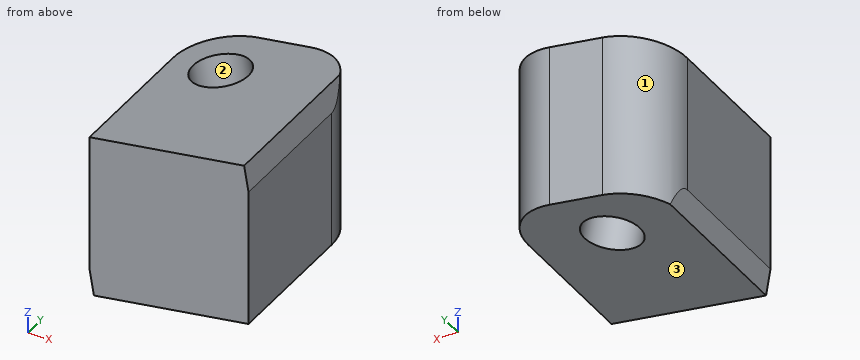
Autodesk Inventor part; units mm, degrees
ref_plane "YZ Plane" through (0, 0, 0) normal (1, 0, 0) x (0, 1, 0)
ref_plane "XZ Plane" through (0, 0, 0) normal (0, 1, 0) x (-1, 0, 0)
ref_plane "XY Plane" through (0, 0, 0) normal (0, 0, 1) x (1, 0, 0)
sketch "BaseSC" plane through (0, 0, 0) normal (0, 1, 0) x (-1, 0, 0)
  line L0 (15, 13) -> (-15, 13)
  line L1 (-15, 13) -> (-15, -13)
  line L2 (-15, -13) -> (15, -13)
  line L3 (15, -13) -> (15, 13)
  line L4 (15, 13) -> (-15, -13) construction
  line L5 (-15, 13) -> (15, -13) construction
  line L6 (15, 13) -> (14.1667, 17.9301)
  line L7 (14.1667, 17.9301) -> (-15, 13)
  line L8 (0, 0) -> (8.3423, 0)
  line L9 (15, -13) -> (14.1667, -17.9301)
  line L10 (14.1667, -17.9301) -> (-15, -13)
  line L11 (-15, 13) -> (-14.1667, 17.9301)
  line L12 (-14.1667, 17.9301) -> (15, 13)
  dimension "d0" = 30
  dimension "d1" = 26
  dimension "d9" = 5
  dimension "d10" = 90
  dimension "d17" = 5
  dimension "d18" = 90
sketch "スケッチ2" plane through (0, 0, 0) normal (0, 0, 1) x (1, 0, 0)
  point P0 (0, 0)
extrude "押し出し1" add sketch "BaseSC" against normal blind 30 contours L3 L2 L1 L0
sketch "スケッチ3" plane through (15, 0, 13) normal (1, 0, 0) x (0, 0, -1)
  line L0 (2.5, -1.5742) -> (23.5, -1.5742)
  line L1 (23.5, -1.5742) -> (23.5, -28.5742)
  line L2 (23.5, -28.5742) -> (2.5, -28.5742)
  line L3 (2.5, -28.5742) -> (2.5, -1.5742)
  line L4 (2.5, -1.5742) -> (23.5, -28.5742) construction
  line L5 (23.5, -1.5742) -> (2.5, -28.5742) construction
  ellipse E0 centre (13, -15.0742) end of major axis (23.5, -15.0742) minor radius 13.5
  point P0 (13, 0)
  dimension "d5" = 21
  dimension "d6" = 27
extrude "押し出し2" cut sketch "スケッチ3" against normal through all contours E0
extrude "押し出し3" add sketch "BaseSC" along normal blind 36 contours L3 L2 L1 L0 | L9 L10 L2
extrude "押し出し5" add sketch "BaseSC" along normal blind 36 contours L0 L7 L12 | L11 L12 L7
sketch "スケッチ5" plane through (-14.1667, 0, -17.9301) normal (0.1666667, 0, -0.9860133) x (-0.9860133, 0, -0.1666667)
  circle A0 centre (-14.1422, 25) radius 5.3
  line L0 (-29.5804, 0) -> (0, 0)
  point P0 (-16.9569, 0)
  dimension "d21" = 10.6
  dimension "d22" = 25
extrude "押し出し6" cut sketch "スケッチ5" against normal through all
sketch "スケッチ6" plane through (0, -30, 0) normal (0, -1, 0) x (1, 0, 0)
  line L0 (15, -1) -> (-15, -1)
  line L1 (-15, -1) -> (-15, 1)
  line L2 (-15, 1) -> (15, 1)
  line L3 (15, 1) -> (15, -1)
  line L4 (15, -1) -> (-15, 1) construction
  line L5 (-15, -1) -> (15, 1) construction
  point P0 (0, 0)
  dimension "d25" = 30
  dimension "d26" = 2
extrude "押し出し7" cut sketch "スケッチ6" against normal blind 5
fillet "フィレット1" radius 10 2 edges at (15, 36, 0) (-15, 36, 0)
sketch "スケッチ7" plane through (-15, -30, 13) normal (0, 0, 1) x (1, 0, 0)
  line L0 (30, 30) -> (0, 30)
  line L1 (0, 0) -> (0, 30)
  line L2 (30, 0) -> (0, 0)
  line L3 (30, 30) -> (30, 0)
  point P0 (15, 30)
extrude "押し出し8" cut sketch "スケッチ7" against normal through all
properties part number "default"
Check sheet for the modelled part. Datum: model origin and axes. Units: mm. Face numbers are marked on the shaded views. Round coordinates to 2 decimals unless told otherwise and drop trailing zeros. Order: outer loops, then holes, each group sorted by start corner. A loop starts at its lowest first (then second) coordinate and runs counter-clockwise, first axis right, second up.
1) Section check D-D (y = 31). Record the boundary of the cut face in (x, z), and give its area (3 significant figures).
2) Section check A-A (y = 23). Record the boundary of the cut face in (x, z), and give its area (3 significant figures).
3) Mould release check, pull along X, two halves, no side actions. Record for the marked faces 1, 2 and 3: +X half, -X half, draft (parallel to the pull), parting line (faces both ways), or undercut.
4) Scan lines: line 1 (X direction, y = 20.5, z = -0.5); line 2 (X direction, y = 28, z = 10); line 3 (Y direction, x = 3.5, z = -11.5). Record each from-to range of solid material in increasing order.
5) Go/stop test with flat-tipped pins: pin 1 Ø1 at (x, y) = (-0.5, 3.5) entering from -Z; pin 2 Ø12 at (x, y) = (11.5, 6.5) entering from +Z; pin 3 Ø5 at (x, y) = (-1, 14.5) entering from -Z. Record where each tip stops, or that it passes through.
6) Section check B-B (y = 5). Record the boundary of the cut face in (x, z).
7) Section check C-C (x = 12). Record the boundary of the cut face in (y, z).
Result:
1. outline: (-13.66, -17.84) - (13.66, -13.23) - (13.66, 17.84) - (-13.66, 13.23) - close
1. area: 849 mm2
2. outline: (-15, -13) - (-14.17, -17.93) - (-5.06, -16.39) - (-10.17, 13.82) - (-15, 13) - close; (-0.49, 15.45) - (4.62, -14.76) - (15, -13) - (15, 13) - (14.17, 17.93) - close
2. area: 627 mm2
3. face 1: -X half
3. face 2: undercut
3. face 3: +X half
4. line 1: x = -15 to -5.61, 0.07 to 15
4. line 2: x = -14.8 to -8.98, -0.11 to 14.8
4. line 3: y = 0 to 21.97, 28.03 to 36
5. pin 1: stops at z = -15.7
5. pin 2: stops at z = 17.93
5. pin 3: stops at z = -16.13
6. outline: (-15, -13) - (-14.17, -17.93) - (15, -13) - (15, 13) - (14.17, 17.93) - (-15, 13) - close
7. outline: (0, -13.51) - (33.14, -13.51) - (33.14, 17.56) - (0, 17.56) - close
